Part model, mm, in its own coordinate system. Give positions to 0.01 mm unless a question says otherwise; leave off trailing zeros. Order: outer loops, then holes, each group sorted by start corner. A loop starts at its lowest first (then second) coordinate and runs counter-clockwise, first axis right, second up. Notation, with made-up numbers: (73.25, 2) - (93.25, 2) arc R24 cw to (93.25, 28) - close; hole circle Ø7 at (69, 47). An arc over 180 degrees is marked (long way). One line per item, written item: value.
Autodesk Inventor part; units mm, degrees
ref_plane "YZ Plane" through (0, 0, 0) normal (1, 0, 0) x (0, 1, 0)
ref_plane "XZ Plane" through (0, 0, 0) normal (0, 1, 0) x (-1, 0, 0)
ref_plane "XY Plane" through (0, 0, 0) normal (0, 0, 1) x (1, 0, 0)
sketch "Szkic8" plane through (0, 0, 0) normal (0, 1, 0) x (-1, 0, 0)
  circle A0 centre (0, 0) radius 31.75
  circle A1 centre (0, 0) radius 30.55
  dimension "d53" = 63.5
  dimension "d54" = 1.2
extrude "Wyciągnięcie proste2" add sketch "Szkic8" along normal mid plane 210
sketch "Szkic13" plane through (0, 0, 0) normal (0, 0, 1) x (1, 0, 0)
  circle A0 centre (0, 0) radius 12.5
  circle A1 centre (0, 0) radius 11.3
  dimension "d67" = 25
  dimension "d68" = 1.2
extrude "Wyciągnięcie proste6" add sketch "Szkic13" along normal blind 35
sketch "Szkic14" plane through (0, 0, 35) normal (0, 0, 1) x (1, 0, 0)
  circle A0 centre (0, 0) radius 11.3
extrude "Wyciągnięcie proste7" cut sketch "Szkic14" against normal blind 35
sketch "Szkic15" plane through (0, -105, 0) normal (0, -1, 0) x (1, 0, 0)
  circle A0 centre (0, 0) radius 30.55
extrude "Wyciągnięcie proste8" cut sketch "Szkic15" against normal blind 210
fillet "Zaokrąglenie3" radius 1.2 2 edges at (-0.0043, 12.5, 31.75) (0.003, -12.5, 31.75)
fillet "Zaokrąglenie4" radius 2.4 2 edges at (-0.002, -11.3, 30.55) (-0.0004, 11.3, 30.55)
equation "\"d53\" = OD"
equation "\"d54\" = THK"
equation "\"d55\" = L1"
equation "\"d67\" = OD2"
equation "\"d68\" = THK"
equation "\"d69\" = L2"
equation "\"d71\" = L2"
equation "\"d73\" = L1"
equation "\"d75\" = THK"
equation "\"d76\" = 2 * THK"
equation "\"SzerokośćGięciaPodcięcia\" = Grubość"
equation "\"RozmiarPodcięciaNarożnika\" = 4 * Grubość"
equation "\"PromieńPrzejścia\" = PromieńGięcia"
equation "\"Rozmiar_promienia_Jacobiego\" = PromieńGięcia"
equation "\"Wielk_odstępu\" = Grubość"
equation "\"d2\" = PromieńGięcia"
equation "\"d23\" = PromieńGięcia"
equation "\"OD\" = 63.5"
equation "\"THK\" = 1.2"
equation "\"L1\" = 210"
equation "\"L2\" = 35"
equation "\"OD2\" = 25"
properties part number "Trójnik red. krótki  Ø63,5 25 63,5 s=1,2 L=210" material "304"
1) Drill centre lines: line 1 along X through (y, z) = (0, 33.5); line 2 along Z through (x, y) = (0, 43.5); line 3 along X through (y, z) = (24.5, 1). Where is each one in solid material? Low to high. Write a range as from..to.
Outcome:
line 1: x = -12.5..-11.3, 11.3..12.5
line 2: z = -31.75..-30.55, 30.55..31.75
line 3: x = -31.73..-30.53, 30.53..31.73
2) Cut at B-B, the plane x = -16. Give the cut face in (y, z).
Outcome:
outline: (-105, -27.42) - (105, -27.42) - (105, -26.03) - (-105, -26.03) - close; (-105, 26.03) - (105, 26.03) - (105, 27.42) - (-105, 27.42) - close
3) Cut at C-C, the plane x = 0. Give the number of separate pieces and of enclosed holes in the cut face, then the cut area to 3 significant figures.
Outcome:
separate pieces: 3
enclosed holes: 0
area: 483 mm^2
4) Cut at D-D, the plane y = -79. Give the cut face in (x, z).
Outcome:
outline: circle Ø63.5 at (0, 0); hole circle Ø61.1 at (0, 0)
5) Pin check, flat tips, straight feed: pin 1 (1.5 mm diameter, centred on y = 27.5, z = -12.5, fed in from -X); pin 2 (8 mm diameter, centred on y = 25.5, z = 17, fed in from -X); pin 3 (1.5 mm diameter, centred on x = -6.5, y = 42.5, fed in from -Z) (3 decimals). Stop position of each tip, or through.
Outcome:
pin 1: stops at x = -29.5
pin 2: stops at x = -28.97
pin 3: stops at z = -31.225
6) Mould opens along X. For faces 1 (the cylindrical face through (-2.71, 12.203, 33.007)), 2 (the cylindrical face through (-14.1, 1.5, -27.1)), 3 (the cylindrical face through (-2.45, 11.03, 33.01)), 4 (the flat face through (17, -105, 26)) say: released by +X, released by -X, zero draft, split by the parting line, or undercut.
Outcome:
face 1: split by the parting line
face 2: undercut
face 3: undercut
face 4: zero draft
7) Cut at A-A, the plane z = 0. Give the cut face in (x, y).
Outcome:
outline: (-31.75, -105) - (-30.55, -105) - (-30.55, 105) - (-31.75, 105) - close; (30.55, -105) - (31.75, -105) - (31.75, 105) - (30.55, 105) - close
